Autodesk Inventor part; units mm, degrees
ref_plane "作業平面1" through (-53.8577, -21, 178) normal (0, 0, -1) x (0, 1, 0)
ref_plane "YZ Plane" through (0, 0, 0) normal (1, 0, 0) x (0, 1, 0)
ref_plane "XZ Plane" through (0, 0, 0) normal (0, 1, 0) x (-1, 0, 0)
sketch "スケッチ1" plane through (0, 0, 0) normal (0, 0, 1) x (1, 0, 0)
  line L0 (-53.8577, -21) -> (53.8577, -21)
  line L1 (53.8577, -21) -> (53.8577, 21)
  line L2 (53.8577, 21) -> (48.8577, 21)
  line L3 (48.8577, 21) -> (49.7747, 18.6743)
  line L4 (49.7747, 18.6743) -> (-44.506, -18.5)
  line L5 (-44.506, -18.5) -> (-45.423, -16.1743)
  line L6 (-45.423, -16.1743) -> (-53.8577, -19.5)
  line L7 (-53.8577, -19.5) -> (-53.8577, -21)
  line L8 (-14.7433, -12.1394) -> (42.0411, 10.2503)
  arc A0 (44.7747, 8.3897) -> (42.0411, 10.2503) centre (42.7747, 8.3897) ccw
  line L9 (44.7747, 8.3897) -> (44.7747, -14)
  arc A1 (42.7747, -16) -> (44.7747, -14) centre (42.7747, -14) ccw
  line L10 (42.7747, -16) -> (-14.0097, -16)
  arc A2 (-14.7433, -12.1394) -> (-14.0097, -16) centre (-14.0097, -14) ccw
  line L11 (49.7747, 18.6743) -> (53.8577, 18.6743)
  point P0 (0, 0)
ref_plane "作業平面1" through (-53.8577, -21, 178) normal (0, 0, -1) x (0, 1, 0)
extrude "押し出し1" add sketch "スケッチ1" along normal up to surface (178 mm away) contours L11 L3 L2 L1
ref_plane "作業平面2" through (53.8577, 21, -10) normal (-1, 0, 0) x (0, 1, 0)
sketch "スケッチ3" plane through (53.8577, 21, -10) normal (-1, 0, 0) x (0, 1, 0)
  line L0 (-2.3257, -10) -> (-2.3257, -188)
  line L1 (-2.3257, -10) -> (0, -10)
  line L2 (-2.3257, -10) -> (-10.3257, -10)
  line L3 (-10.3257, -10) -> (-10.3257, -18)
  line L4 (-10.3257, -18) -> (-2.3257, -18)
  line L5 (-2.3257, -18) -> (-2.3257, -10)
  circle A0 centre (-6.3257, -14) radius 1.5
  line L6 (-3.4757, -15.6454) -> (-6.3257, -17.2909)
  line L7 (-6.3257, -17.2909) -> (-9.1757, -15.6454)
  line L8 (-9.1757, -15.6454) -> (-9.1757, -12.3546)
  line L9 (-9.1757, -12.3546) -> (-6.3257, -10.7091)
  line L10 (-6.3257, -10.7091) -> (-3.4757, -12.3546)
  line L11 (-3.4757, -12.3546) -> (-3.4757, -15.6454)
  point P0 (-21, -10)
  dimension "d5" = 8
  dimension "d6" = 8
  dimension "d7" = 3
  dimension "d8" = 5.7
extrude "押し出し2" add sketch "スケッチ3" along normal blind 4.083 contours L0 L4 L3 L2 | L6 L7 L8 L9 L10 L11
ref_plane "作業平面4" through (49.7747, 18.6743, 0) normal (1, 0, 0) x (0, 0, -1)
sketch "スケッチ4" plane through (49.7747, 21, -10) normal (-1, 0, 0) x (0, 0, 1)
  circle A0 centre (14, -6.3257) radius 1.5
  line L0 (12.3546, -9.1757) -> (10.7091, -6.3257)
  line L1 (10.7091, -6.3257) -> (12.3546, -3.4757)
  line L2 (12.3546, -3.4757) -> (15.6454, -3.4757)
  line L3 (15.6454, -3.4757) -> (17.2909, -6.3257)
  line L4 (17.2909, -6.3257) -> (15.6454, -9.1757)
  line L5 (15.6454, -9.1757) -> (12.3546, -9.1757)
  point P0 (10, -21)
  point P1 (14, -3.4757)
  point P2 (14, -9.1757)
  dimension "d11" = 5.7
extrude "押し出し3" cut sketch "スケッチ4" against normal blind 3
sketch "スケッチ5" plane through (49.7747, 21, -10) normal (-1, 0, 0) x (0, 0, 1)
  line L0 (18, -2.3257) -> (10, -2.3257)
  line L1 (18, -2.3257) -> (188, -2.3257)
  line L2 (18, -10.3257) -> (18, -2.3257)
  line L3 (18, -2.3257) -> (21, -2.3257)
  line L4 (21, -2.3257) -> (21, -5.3257)
  line L5 (21, -5.3257) -> (18, -5.3257)
  line L6 (18, -5.3257) -> (18, -2.3257)
  arc A0 (21, -2.3257) -> (18, -5.3257) centre (21, -5.3257) ccw
  point P0 (10, -21)
  point P1 (21, -2.3257)
  dimension "d14" = 3
  dimension "d15" = 3
extrude "押し出し4" add sketch "スケッチ5" against normal blind 4.083 contours L1 A0 L2
ref_plane "作業平面5" through (48.8577, 21, 89) normal (0, 0, 1) x (1, 0, 0)
mirror "ミラー1" about plane through (48.8577, 21, 89) normal (0, 0, 1) of "押し出し2", "押し出し4"
mirror "ミラー2" about plane through (48.8577, 21, 89) normal (0, 0, 1) of "押し出し3"
ref_plane "作業平面6" through (48.8577, 21, 89) normal (0, 0, 1) x (1, 0, 0)
equation "\"d6\" = d5"
properties part number "Spcer_Upper"
Input: part model. Units: mm. Frame: model coordinates. A direction names the side the tool comes from. Coordinates: 2 decimals unless noted, no trailing zeros. Loops run counter-clockwise (first coordinate to the right, second up) from the corner with the lowest first, then second, coordinate; pieces in that order, holes last. Notation, with made-up numbers: M 31,60 L 46,60 A34 cw 46,99 Z; hole C -22.75,-25 d1. An arc over 180 degrees is marked long. One line per item, written item: value.
(1) Line query: line 1 along Z through (x, y) = (50.05, 14.25); line 2 along Z through (x, y) = (52.2, 15.5); line 3 along Y through (x, z) = (50.5, 67.5). Output: solid intervals per line, ascending. Write a range as from..to.
Filled in:
line 1: 0..0.95, 7.05..8, 170..170.95, 177.05..178
line 2: 0..1.19, 6.81..8, 170..171.19, 176.81..178
line 3: 18.67..21
(2) Section B-B (z = 30.5). Output: boundary loops of the cut face in (x, y), and give its area (3 significant figures).
Filled in:
outline: M 48.86,21 L 49.77,18.67 L 53.86,18.67 L 53.86,21 Z
area: 10.6 mm^2
(3) Pull-direction query (Y, two-part tool) for faces 1 (the flat face through (52, 16, 178)), 2 (the flat face through (52, 10.674, 4)), 3 (the flat face through (51, 17.524, 4)); classes: +Y half, -Y half, draft (parallel to the pull), parting line (faces both ways), or undercut.
Filled in:
face 1: draft
face 2: -Y half
face 3: undercut
(4) Pin query (flat end, axial travel): pin 1 (4.5 mm diameter, centred on y = 14, z = 173, fed in from -X); pin 2 (2 mm diameter, centred on x = 52, z = 104, fed in from -Y); pin 3 (2.5 mm diameter, centred on y = 14.67, z = 174, fed in from +X); pin 4 (3 mm diameter, centred on y = 15.5, z = 4, fed in from -X). Return the tip coordinate at first contact, or that it passes through.
Filled in:
pin 1: x = 49.77
pin 2: y = 18.67
pin 3: through
pin 4: x = 52.77
(5) Section A-A (z = 4). Output: boundary loops of the cut face in (x, y).
Filled in:
outline: M 48.86,21 L 49.77,18.67 L 49.77,17.52 L 52.77,17.52 L 52.77,16.17 L 53.86,16.17 L 53.86,21 Z; M 49.77,10.67 L 53.86,10.67 L 53.86,13.17 L 52.77,13.17 L 52.77,11.82 L 49.77,11.82 Z
(6) Reachability of faces 4 (the flat face through (51, 17.524, 174)), 5 (the flat face through (52, 10.674, 174)), 6 (the flat face through (52, 13, 170)), 7 (the flat face through (52, 16, 0)), 8 (the flat face through (49.775, 16, 171)) from +Z, -Z, +X, -X, +Y, -Y: full face, straight path, thin tool, end or side. Return the list, or none.
Filled in:
face 4: -X
face 5: +Z, -Z, +X, -X, -Y
face 6: +X, -X, -Y
face 7: -Z, +X, -X, +Y, -Y
face 8: +Z, -Z, -X, -Y
